Build history of the part. All positions in model axes, mm. A direction names the side the tool comes from. Round coordinates to 2 decimals unless told otherwise and drop trailing zeros. Loops run counter-clockwise (first coordinate to the right, second up) from the corner with the lowest first, then second, coordinate; pieces in that order, holes last. Notation, with made-up numbers: (37.25, 47) - (70.25, 47) arc R26 ccw to (70.25, 86) - close; hole circle Ø7 at (-32.75, 16.25). An arc over 180 degrees is marked (long way). Use a Markdown table: item, result.
from build123d import *

# Parameters (mm, degrees)
F0_W     = 84
F0_H     = 75
F1_DEPTH = 2
F2_W     = 84
F2_H     = 75
F2_W_2   = 80
F2_H_2   = 71
F3_DEPTH = 25
F4_W     = 73
F4_H     = 2.1
F5_DEPTH = 83
F6_W     = 71
F6_H     = 20.9
F7_DEPTH = 2


with BuildPart() as f1:
    # F0 (on Top) → F1 (new body)
    with BuildSketch(Plane.XY):
        with Locations((-2.925097, 5.706407)):
            Rectangle(F0_W, F0_H)
    extrude(amount=-F1_DEPTH)

    # F2 (on face) → F3 (join)
    with BuildSketch(Plane.XY):
        with Locations((-2.925097, 5.706407)):
            Rectangle(F2_W, F2_H)
        with Locations((-2.925097, 5.706407)):
            Rectangle(F2_W_2, F2_H_2, mode=Mode.SUBTRACT)
    extrude(amount=F3_DEPTH)

    # F4 (on face) → F5 (cut)
    with BuildSketch(Plane(origin=(-44.925097, 0, 0), x_dir=(0, -1, 0), z_dir=(-1, 0, 0))):
        with Locations((-5.706407, 21.95)):
            Rectangle(F4_W, F4_H)
    extrude(amount=-F5_DEPTH, mode=Mode.SUBTRACT)

    # F6 (on face) → F7 (cut)
    with BuildSketch(Plane(origin=(-44.925097, 0, 0), x_dir=(0, -1, 0), z_dir=(-1, 0, 0))):
        with Locations((-5.706407, 10.45)):
            Rectangle(F6_W, F6_H)
    extrude(amount=-F7_DEPTH, mode=Mode.SUBTRACT)


solid = f1.part
Q1. Cut at A-A, the plane y = 23. List the corners of the cut face in (x, z), plus the area to 3 significant figures.
Results found:
| item | result |
|---|---|
| outline | (-44.93, -2) - (39.07, -2) - (39.07, 25) - (37.07, 25) - (37.07, 23) - (38.07, 23) - (38.07, 20.9) - (37.07, 20.9) - (37.07, 0) - (-44.93, 0) - close; (-44.93, 23) - (-42.93, 23) - (-42.93, 25) - (-44.93, 25) - close |
| area | 220 mm2 |
Q2. Drop flat-ended pins along their axis: pin 1 (1.7 mm diameter, centred on y = -6, z = 22, fed in from -X); pin 2 (1.5 mm diameter, centred on y = 11, z = 9, fed in from -X); pin 3 (12 mm diameter, centred on y = 0.5, z = 3.5, fed in from -X); pin 4 (21.5 mm diameter, centred on x = 6, y = 3.5, fed in from +Z). Give the stop position or say it passes through.
Results found:
| item | result |
|---|---|
| pin 1 | stops at x = 38.07 |
| pin 2 | stops at x = 37.07 |
| pin 3 | stops at x = -44.93 |
| pin 4 | stops at z = 0 |
Q3. Which spindle directions (+Z, -Z, +X, -X, +Y, -Y) get a long thin tool onto all of the face, cutting with end or side? Do faces 1 (the face through (-44, 6, 23)), 2 (the face through (37.075, 5, 10)), 3 (the face through (37.075, 5, 24)). Say none if no direction does.
Results found:
| item | result |
|---|---|
| face 1 | -X |
| face 2 | +Z, -X |
| face 3 | +Z |
Q4. Probe line 1 (Y direction, x = -36.5, z = 22.25); line 2 (Y direction, x = 7, z = 1.5); line 3 (X direction, y = 39, z = 23.75). List the from-to ranges inside material, lowest first.
Results found:
| item | result |
|---|---|
| line 1 | y = -31.79 to -30.79, 42.21 to 43.21 |
| line 2 | y = -31.79 to -29.79, 41.21 to 43.21 |
| line 3 | x = -44.93 to -42.93, 37.07 to 39.07 |
Q5. Cut at C-C, the plane z = 9.75. List the corners of the cut face in (x, y).
Results found:
| item | result |
|---|---|
| outline | (-44.93, -31.79) - (39.07, -31.79) - (39.07, 43.21) - (-44.93, 43.21) - (-44.93, 41.21) - (37.07, 41.21) - (37.07, -29.79) - (-44.93, -29.79) - close |
Q6. Pull direction Y, two halves, no side cores. Call faces 4 (the face through (-44.925, 2.8, 23.4)), 5 (the face through (-4, 43.206, 11)), 6 (the face through (-4, 42.206, 22)): pulls with the +Y half, pulls with the -Y half, needs draft (parallel to the pull), parting line crosses it, or undercut.
Results found:
| item | result |
|---|---|
| face 4 | needs draft |
| face 5 | pulls with the +Y half |
| face 6 | undercut |
Q7. Cut at B-B, the plane x = -5. List the corners of the cut face in (y, z).
Results found:
| item | result |
|---|---|
| outline | (-31.79, -2) - (43.21, -2) - (43.21, 25) - (41.21, 25) - (41.21, 23) - (42.21, 23) - (42.21, 20.9) - (41.21, 20.9) - (41.21, 0) - (-29.79, 0) - (-29.79, 20.9) - (-30.79, 20.9) - (-30.79, 23) - (-29.79, 23) - (-29.79, 25) - (-31.79, 25) - close |
